```python
from build123d import *

# Parameters (mm, degrees)
SKETCH1_W             = 25.4
SKETCH1_H             = 9.525
BOSS_EXTRUDE1_DEPTH   = 106.68
BOSS_EXTRUDE2_DEPTH   = 213.36
CHAMFER1_SIZE         = 6.35
CHAMFER2_SIZE         = 3.175
CHAMFER2_SIZE2        = 2.93072295
F_8_CLEARANCE_HOLE1_D = 4.9149
CHAMFER3_SIZE         = 1.5875
BOSS_EXTRUDE3_DEPTH   = 3.429
SKETCH6_W             = 15.367
SKETCH6_H             = 20.192862299
SKETCH6_R             = 2.45745
BOSS_EXTRUDE4_DEPTH   = 3.175
SKETCH7_R             = 6.35
BOSS_EXTRUDE5_DEPTH   = 6.604
CUT_EXTRUDE1_DEPTH    = 218.112793351


with BuildPart() as part:
    # Sketch1 → Boss-Extrude1 (new, symmetric)
    with BuildSketch(Plane(origin=(0, 0, 0), x_dir=(0, 0, -1), z_dir=(1, 0, 0))):
        Rectangle(SKETCH1_W, SKETCH1_H)
    extrude(amount=BOSS_EXTRUDE1_DEPTH, both=True)

    # Sketch2 → Boss-Extrude2 (add, through all)
    with BuildSketch(Plane.ZY.offset(106.68)):
        Polygon((12.7, 4.7625), (37.438033761, 4.7625), (38.828997162, -11.13628443), (12.7, -11.13628443), align=None)
    extrude(amount=-BOSS_EXTRUDE2_DEPTH)

    # Chamfer1
    chamfer1_edges = [part.edges().sort_by_distance(p)[0] for p in [
        (106.68, 0, -12.7),
        (106.68, -7.949392215, 12.7),
        (-106.68, -7.949392215, 12.7),
        (-106.68, 0, -12.7),
    ]]
    chamfer(chamfer1_edges, length=CHAMFER1_SIZE)

    # Chamfer2
    chamfer2_edges = [part.edges().sort_by_distance(p)[0] for p in [
        (0, -11.13628443, 38.828997162),
    ]]
    chamfer2_side = [part.faces().sort_by_distance(p)[0] for p in [
        (0, -3.186892215, 38.133515462),
    ]]
    chamfer(chamfer2_edges, length=CHAMFER2_SIZE, length2=CHAMFER2_SIZE2, reference=chamfer2_side[0])

    # #8 Clearance Hole1 (through all)
    with Locations(Plane(origin=(0, -11.13628443, 0), x_dir=(-1, 0, 0), z_dir=(0, -1, 0))):
        with Locations((-81.28, -25.62613884), (0, 0), (0, -25.62613884), (81.28, -25.62613884), (81.28, 0), (-81.28, 0)):
            Hole(F_8_CLEARANCE_HOLE1_D / 2)

    # Chamfer3
    chamfer3_edges = [part.edges().sort_by_distance(p)[0] for p in [
        (0, -11.13628443, 12.7),
        (-106.68, -11.13628443, 27.474137106),
        (106.68, -11.13628443, 27.474137106),
        (-103.505, -11.13628443, 15.875),
        (103.505, -11.13628443, 15.875),
        (0, -4.7625, -12.7),
        (-103.505, -4.7625, -9.525),
        (103.505, -4.7625, -9.525),
        (-106.68, -4.7625, 6.35),
        (106.68, -4.7625, 6.35),
    ]]
    chamfer(chamfer3_edges, length=CHAMFER3_SIZE)

    # Sketch5 → Boss-Extrude3 (add)
    with BuildSketch(Plane(origin=(0, 4.7625, 0), x_dir=(1, 0, 0), z_dir=(0, 1, 0))):
        Polygon((85.7885, -37.438033761), (85.7885, -23.023155151), (81.28, -20.420171462), (76.7715, -23.023155151), (76.7715, -37.438033761), (73.5965, -37.438033761), (73.5965, -17.245171462), (88.9635, -17.245171462), (88.9635, -37.438033761), align=None)
        Polygon((4.5085, -37.438033761), (4.5085, -23.023155151), (0, -20.420171462), (-4.5085, -23.023155151), (-4.5085, -37.438033761), (-7.6835, -37.438033761), (-7.6835, -17.245171462), (7.6835, -17.245171462), (7.6835, -37.438033761), align=None)
        Polygon((-76.7715, -37.438033761), (-76.7715, -23.023155151), (-81.28, -20.420171462), (-85.7885, -23.023155151), (-85.7885, -37.438033761), (-88.9635, -37.438033761), (-88.9635, -17.245171462), (-73.5965, -17.245171462), (-73.5965, -37.438033761), align=None)
    extrude(amount=BOSS_EXTRUDE3_DEPTH)

    # Sketch6 → Boss-Extrude4 (add)
    with BuildSketch(Plane(origin=(0, 8.1915, 0), x_dir=(1, 0, 0), z_dir=(0, 1, 0))):
        with Locations((-81.28, -27.341602612)):
            Rectangle(SKETCH6_W, SKETCH6_H)
        with Locations(Location((-81.28, -25.62613884, 0), (0, 0, 90))):
            Circle(SKETCH6_R, mode=Mode.SUBTRACT)
        with Locations((0, -27.341602612)):
            Rectangle(SKETCH6_W, SKETCH6_H)
        with Locations(Location((0, -25.62613884, 0), (0, 0, 90))):
            Circle(SKETCH6_R, mode=Mode.SUBTRACT)
        with Locations((81.28, -27.341602612)):
            Rectangle(SKETCH6_W, SKETCH6_H)
        with Locations(Location((81.28, -25.62613884, 0), (0, 0, 90))):
            Circle(SKETCH6_R, mode=Mode.SUBTRACT)
    extrude(amount=BOSS_EXTRUDE4_DEPTH)

    # Sketch7 → Boss-Extrude5 (add)
    with BuildSketch(Plane(origin=(0, 4.7625, 0), x_dir=(1, 0, 0), z_dir=(0, 1, 0))):
        Polygon((-73.5965, -17.245171462), (-73.5965, -37.438033761), (-7.6835, -37.438033761), (-7.6835, -17.245171462), (7.6835, -17.245171462), (7.6835, -37.438033761), (73.5965, -37.438033761), (73.5965, -17.245171462), (88.9635, -17.245171462), (88.9635, -37.438033761), (106.68, -37.438033761), (106.68, 6.35), (100.33, 12.7), (-100.33, 12.7), (-106.68, 6.35), (-106.68, -37.438033761), (-88.9635, -37.438033761), (-88.9635, -17.245171462), align=None)
        with Locations(Location((81.28, 0, 0), (0, 0, 90))):
            Circle(SKETCH7_R, mode=Mode.SUBTRACT)
        with Locations(Location((0, 0, 0), (0, 0, 90))):
            Circle(SKETCH7_R, mode=Mode.SUBTRACT)
        with Locations(Location((-81.28, 0, 0), (0, 0, 90))):
            Circle(SKETCH7_R, mode=Mode.SUBTRACT)
    extrude(amount=BOSS_EXTRUDE5_DEPTH)

    # Sketch8 → Cut-Extrude1 (cut, through all)
    with BuildSketch(Plane.ZY.offset(106.68)):
        Polygon((37.438033761, 4.7625), (36.860258627, 11.3665), (37.438033761, 11.3665), align=None)
    extrude(amount=-CUT_EXTRUDE1_DEPTH, mode=Mode.SUBTRACT)


solid = part.part
```
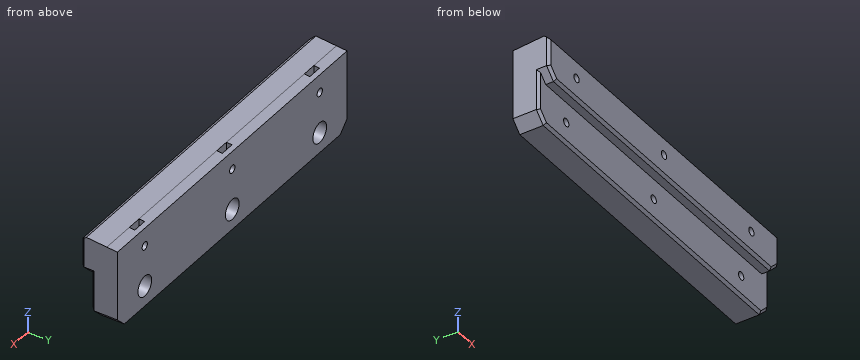
Design review of the part built by this model. Coordinates are the model's own, in mm. Coordinates: 2 decimals unless noted, no trailing zeros. Write each loop counter-clockwise with the first axis right and the second up, starting at its lowest first coordinate (ties: lowest second). Pieces come first, ordered by that corner, then holes.
1) Add section C-C (y = 2.75). Write out the cut boundary in (x, z), plus the area to 3 significant figures.
2) To check wall thickness, follow L1, parallel to X at y = 5.25, z = 30.5; L2, parallel to X at y = 8, z = 0; L3, parallel to Z at x = 81.28, y = 8.25. State the ranges of each line that lie inside material, in increasing order.
3) Insertion check: pin 1 (3 mm diameter, centred on x = -81.28, z = 25.63, fed in from +Y); pin 2 (10 mm diameter, centred on x = -81.28, z = 0, fed in from -Y); pin 3 (8 mm diameter, centred on x = -32.5, y = -2.5, fed in from +Z). Each pin has a flat end and moves straight along its axis. Give the tip position at first contact, or say it passes through.
4) Add section B-B (x = -54). Write out the cut boundary in (y, z) (1 decimal), plus the area to 3 significant figures.
5) Add section A-A (z = 0). State how many separate pieces and enclosed holes the cut face has, plus the area to 3 significant figures.
6) Add section D-D (z = 9.5). Write out the cut boundary in (x, y) (1 decimal), plus the area to 3 significant figures.
Check result:
1. outline: (-106.68, -6.35) - (-100.33, -12.7) - (100.33, -12.7) - (106.68, -6.35) - (106.68, 37.61) - (-106.68, 37.61) - close; hole circle Ø4.91 at (-81.28, 0); hole circle Ø4.91 at (-81.28, 25.63); hole circle Ø4.91 at (0, 0); hole circle Ø4.91 at (0, 25.63); hole circle Ø4.91 at (81.28, 0); hole circle Ø4.91 at (81.28, 25.63)
1. area: 10,600 mm2
2. L1: x = -106.68 to -85.79, -76.77 to -4.51, 4.51 to 76.77, 85.79 to 106.68
2. L2: x = -106.68 to -87.63, -74.93 to -6.35, 6.35 to 74.93, 87.63 to 106.68
2. L3: z = -12.7 to -6.35, 6.35 to 23.17, 28.08 to 37.13
3. pin 1: passes through
3. pin 2: stops at y = -4.76
3. pin 3: stops at z = 38.42
4. outline: (-11.1, 14.3) - (-9.5, 12.7) - (-4.8, 12.7) - (-4.8, -11.1) - (-3.2, -12.7) - (11.4, -12.7) - (11.4, 36.9) - (-8, 38.6) - (-11.1, 35.9) - close
4. area: 968 mm2
5. separate pieces: 4
5. enclosed holes: 0
5. area: 3,050 mm2
6. outline: (-106.7, -3.2) - (-105.1, -4.8) - (105.1, -4.8) - (106.7, -3.2) - (106.7, 11.4) - (-106.7, 11.4) - close
6. area: 3,440 mm2
